Geometry check sheet. Reference: the model listing, model coordinates, mm. A direction names the side the tool comes from. Round coordinates to 2 decimals unless told otherwise and drop trailing zeros. Write each loop counter-clockwise with the first axis right and the second up, starting at its lowest first coordinate (ties: lowest second). Pieces come first, ordered by that corner, then holes. Notation, with made-up numbers: M 33,-1.75 L 40,-1.75 A15 cw 40,13.25 Z; hole C 71,32.5 d11. An arc over 180 degrees is marked long. Put each result on its own line as item: value. Start each with the question number.
(1) Section check C-C on x = -1.5. Record the cut outline in (y, z), then the cut area to 3 significant figures.
(2) Section check B-B on y = 0. Count the separate pieces of the cut face and the enclosed holes in it, then the cut area to 3 significant figures.
(3) Gauge pin test, flat ends, axial feed: pin 1 (4 mm diameter, centred on x = -3, z = 14, fed in from +Y); pin 2 (2 mm diameter, centred on x = 1, z = -34, fed in from +Y); pin 3 (8 mm diameter, centred on x = -3.5, z = -48.5, fed in from +Y); pin 4 (7 mm diameter, centred on y = -54.13, z = 31.25, fed in from +X). Record the tip position at first contact, or that the pin passes through.
(4) Mould release check, pull along Y, two halves, no side actions. Record for faces 1 (the cylindrical face through (-0.059, -1.352, 58.208)), 2 (the cylindrical face through (9.18, 15.02, 47.69)), 3 (the flat face through (-4.25, 47.3, -17.1)): pulls with the +Y half, pulls with the -Y half, needs draft (parallel to the pull), parting line crosses it, or undercut.
(5) Section check A-A on z = 0. Record the cut outline in (x, y).
(6) Material ranges on probe 1 along Z at (x, y) = (-2.5, 50); probe 2 along Z at (x, y) = (-3.5, -54.5); probe 3 along Z at (x, y) = (-2, 3.5), recorded low to high.
(7) Section check D-D on x = -9. Record the cut outline in (y, z).
(8) Tool access check on faces 4 (the cylindrical face through (-15.507, 2.11, -47.954)), 5 (the flat face through (4.25, 47.3, -17.1)), 6 (the cylindrical face through (-0.059, -49.734, -30.274)). Record the directions out of +Z, -Z, +X, -X, +Y, -Y that give a thin tool (end or side, any length) a straight path to the whole face; none if there is none.
Solid Edge part; units mm, degrees
sketch "Sketch1" plane through (0, 0, 0) normal (0, -1, 0) x (1, 0, 0)
  line L0 (-4.25, 72.5) -> (-4.25, 50)
  line L1 (-4.25, 50) -> (-14.25, 50)
  line L2 (-14.25, 50) -> (-15, 48)
  line L3 (-15, 48) -> (-16, 48)
  line L4 (-16, 48) -> (-16, 35)
  line L5 (-16, 35) -> (16, 32.5)
  line L6 (16, 48) -> (16, 32.5)
  line L7 (16, 48) -> (15, 48)
  line L8 (15, 48) -> (14.25, 50)
  line L9 (14.25, 50) -> (4.25, 50)
  line L10 (4.25, 50) -> (4.25, 72.5)
  line L11 (4.25, 72.5) -> (-4.25, 72.5)
  dimension "D1" = 15.5
  dimension "D2" = 14.25
  dimension "D3" = 16
revolve "RevolvedProtrusion1" add sketch "Sketch1" angle 360 about axis through (-60, 0, 0) along (1, 0, 0)
hole "Hole1" at (-4.25, 0, -62.5) direction (1, 0, 0) diameter 9 end up to next
pattern_circular "Pattern1" count 6 over 360 about axis through (-4.25, 0, 0) along (-1, 0, 0) of "Hole1"
extrude "Cutout1" [suppressed]
hole "Bohrung_9" [suppressed]
properties material "Stahl"
Answers follow:
1. outline: C 0,0 d145; hole C -54.13,-31.25 d9; hole C -54.13,31.25 d9; hole C 0,0 d67.73; hole C 0,-62.5 d9; hole C 0,62.5 d9; hole C 54.13,-31.25 d9; hole C 54.13,31.25 d9
1. area: 12,500 mm^2
2. separate pieces: 4
2. enclosed holes: 0
2. area: 1,260 mm^2
3. pin 1: stops at y = 71.5
3. pin 2: stops at y = 64.55
3. pin 3: stops at y = 57.24
3. pin 4: passes through
4. face 1: undercut
4. face 2: parting line crosses it
4. face 3: needs draft
5. outline: M -16,-48 L -15,-48 L -14.25,-50 L -4.25,-50 L -4.25,-72.5 L 4.25,-72.5 L 4.25,-50 L 14.25,-50 L 15,-48 L 16,-48 L 16,-32.5 L -16,-35 Z; M -16,35 L 16,32.5 L 16,48 L 15,48 L 14.25,50 L 4.25,50 L 4.25,72.5 L -4.25,72.5 L -4.25,50 L -14.25,50 L -15,48 L -16,48 Z
6. probe 1: z = -52.5 to -33.04, -29.46 to 29.46, 33.04 to 52.5
6. probe 2: z = -47.81 to -35.73, -26.77 to 26.77, 35.73 to 47.81
6. probe 3: z = -72.42 to -65.33, -59.67 to -33.73, 33.73 to 59.67, 65.33 to 72.42
7. outline: C 0,0 d100; hole C 0,0 d68.91
8. face 4: -X
8. face 5: +X
8. face 6: +X, -X
